The model under review builds one solid part; all positions refer to its coordinate system, in mm. A direction names the side the tool comes from. Give positions to 0.01 mm unless a question says otherwise; leave off trailing zeros. Order: outer loops, then holes, each group sorted by start corner. A loop starts at its lowest first (then second) coordinate and runs counter-clockwise, first axis right, second up. Notation, with made-up numbers: (26.25, 66.25) -> (33.25, 66.25) arc R27 ccw to (33.25, 89.25) -> close; hole circle Ø8 at (2, 19). An arc over 180 degrees is marked (long way). Use one line per item in the form item = value.
```python
from build123d import *

# Parameters (mm, degrees)
SKETCH1_W           = 70
SKETCH1_H           = 20
BOSS_EXTRUDE2_DEPTH = 3
SKETCH3_W           = 3
SKETCH3_H           = 20
BOSS_EXTRUDE3_DEPTH = 18
SKETCH4_W           = 46
SKETCH4_H           = 20
BOSS_EXTRUDE4_DEPTH = 3
SKETCH5_W           = 40
SKETCH5_H           = 3
CUT_EXTRUDE2_DEPTH  = 47.914816423
SKETCH6_R           = 3.1
CUT_EXTRUDE3_DEPTH  = 43.023802779
FILLET2_R           = 3
SKETCH7_R           = 1.6
CUT_EXTRUDE4_DEPTH  = 44.600458713
CUT_EXTRUDE5_DEPTH  = 26
SKETCH10_W          = 46
SKETCH10_H          = 20
BOSS_EXTRUDE5_DEPTH = 3
SKETCH11_R          = 3.1
CUT_EXTRUDE6_DEPTH  = 3
FILLET3_R           = 3


with BuildPart() as part:
    # Sketch1 → Boss-Extrude2 (new body)
    with BuildSketch(Plane(origin=(0, 0, 0), x_dir=(1, 0, 0), z_dir=(0, 1, 0))):
        Rectangle(SKETCH1_W, SKETCH1_H)
    extrude(amount=BOSS_EXTRUDE2_DEPTH)

    # Sketch3 → Boss-Extrude3 (add)
    with BuildSketch(Plane(origin=(0, 3, 0), x_dir=(1, 0, 0), z_dir=(0, 1, 0))):
        with Locations((21.5, 0)):
            Rectangle(SKETCH3_W, SKETCH3_H)
        with Locations((-21.5, 0)):
            Rectangle(SKETCH3_W, SKETCH3_H)
    extrude(amount=BOSS_EXTRUDE3_DEPTH)

    # Sketch4 → Boss-Extrude4 (add)
    with BuildSketch(Plane(origin=(0, 21, 0), x_dir=(1, 0, 0), z_dir=(0, 1, 0))):
        Rectangle(SKETCH4_W, SKETCH4_H)
    extrude(amount=BOSS_EXTRUDE4_DEPTH)

    # Sketch5 → Cut-Extrude2 (cut, through all)
    with BuildSketch(Plane.XY.offset(10)):
        with Locations((0, 1.5)):
            Rectangle(SKETCH5_W, SKETCH5_H)
    extrude(amount=-CUT_EXTRUDE2_DEPTH, mode=Mode.SUBTRACT)

    # Sketch6 → Cut-Extrude3 (cut, through all)
    with BuildSketch(Plane.XZ.offset(-21)):
        with Locations(Location((0, 0, 0), (0, 0, 270))):
            Circle(SKETCH6_R)
    extrude(amount=-CUT_EXTRUDE3_DEPTH, mode=Mode.SUBTRACT)

    # Fillet2
    fillet2_edges = [part.edges().sort_by_distance(p)[0] for p in [
        (-23, 24, 0),
        (23, 24, 0),
        (35, 1.5, 10),
        (-35, 1.5, 10),
        (-35, 1.5, -10),
        (35, 1.5, -10),
    ]]
    fillet(fillet2_edges, radius=FILLET2_R)

    # Sketch7 → Cut-Extrude4 (cut, through all)
    with BuildSketch(Plane.XZ):
        with Locations(Location((-27.499620905, -0.010826829, 0), (0, 0, 270))):
            Circle(SKETCH7_R)
        with Locations(Location((27.500379095, -0.010826829, 0), (0, 0, 270))):
            Circle(SKETCH7_R)
    extrude(amount=-CUT_EXTRUDE4_DEPTH, mode=Mode.SUBTRACT)

    # Sketch9 → Cut-Extrude5 (cut)
    with BuildSketch(Plane.XY.offset(10)):
        Polygon((0, 15.5), (-23, 15.5), (-23, 32.171258166), (25.72707431, 32.171258166), (25.72707431, 15.5), align=None)
    extrude(amount=-CUT_EXTRUDE5_DEPTH, mode=Mode.SUBTRACT)


with BuildPart() as cut_extrude5_piece_1:
    # of the separate pieces the step leaves, piece 1, a body of its own (cut_extrude5_pieces)
    add(part.part.solids().sort_by_distance((20, 15.5, 10))[0])



with BuildPart() as cut_extrude5_piece_2:
    # of the separate pieces the step leaves, piece 2, a body of its own (cut_extrude5_pieces)
    add(part.part.solids().sort_by_distance((-32, 0, 10))[0])


with BuildPart() as cut_extrude5_piece_1_1:
    add(cut_extrude5_piece_1.part)

    add(cut_extrude5_piece_2.part)  # Boss-Extrude5 merges Cut-Extrude5 piece 2
    # Sketch10 → Boss-Extrude5 (add)
    with BuildSketch(Plane(origin=(0, 15.5, 0), x_dir=(1, 0, 0), z_dir=(0, 1, 0))):
        Rectangle(SKETCH10_W, SKETCH10_H)
    extrude(amount=BOSS_EXTRUDE5_DEPTH)

    # Sketch11 → Cut-Extrude6 (cut)
    with BuildSketch(Plane(origin=(0, 18.5, 0), x_dir=(1, 0, 0), z_dir=(0, 1, 0))):
        with Locations(Location((0, 0, 0), (0, 0, 270))):
            Circle(SKETCH11_R)
    extrude(amount=-CUT_EXTRUDE6_DEPTH, mode=Mode.SUBTRACT)

    # Fillet3
    fillet3_edges = [cut_extrude5_piece_1_1.edges().sort_by_distance(p)[0] for p in [
        (-23, 18.5, 0),
        (23, 18.5, 0),
    ]]
    fillet(fillet3_edges, radius=FILLET3_R)


solid = cut_extrude5_piece_1_1.part
```
1. Add section D-D on z = 4.25. Give the boundary of the cut face in (x, y), then the cut area to 3 significant figures.
Values:
outline = (-35, 0) -> (-20, 0) -> (-20, 15.5) -> (20, 15.5) -> (20, 0) -> (35, 0) -> (35, 3) -> (23, 3) -> (23, 15.5) arc R3 ccw to (20, 18.5) -> (-20, 18.5) arc R3 ccw to (-23, 15.5) -> (-23, 3) -> (-35, 3) -> close
area = 299 mm^2
2. Add section B-B on x = 0. Give the boundary of the cut face in (y, z), then the cut area to 3 significant figures.
Values:
outline = (15.5, -10) -> (18.5, -10) -> (18.5, -3.1) -> (15.5, -3.1) -> close; (15.5, 3.1) -> (18.5, 3.1) -> (18.5, 10) -> (15.5, 10) -> close
area = 41.4 mm^2
3. Add section A-A on y = 6.75. Give the boundary of the cut face in (x, z).
Values:
outline = (-23, -10) -> (-20, -10) -> (-20, 10) -> (-23, 10) -> close; (20, -10) -> (23, -10) -> (23, 10) -> (20, 10) -> close
4. Add section C-C on z = 0. Give the boundary of the cut face in (x, y), then the cut area to 3 significant figures.
Values:
outline = (-35, 0) -> (-29.1, 0) -> (-29.1, 3) -> (-35, 3) -> close; (-25.9, 0) -> (-20, 0) -> (-20, 15.5) -> (-3.1, 15.5) -> (-3.1, 18.5) -> (-20, 18.5) arc R3 ccw to (-23, 15.5) -> (-23, 3) -> (-25.9, 3) -> close; (3.1, 15.5) -> (20, 15.5) -> (20, 0) -> (25.9, 0) -> (25.9, 3) -> (23, 3) -> (23, 15.5) arc R3 ccw to (20, 18.5) -> (3.1, 18.5) -> close; (29.1, 0) -> (35, 0) -> (35, 3) -> (29.1, 3) -> close
area = 261 mm^2
5. The part is to be moulded in two halves that separate along X. For faces 1 (the face through (-28.47, 1.48, 1.26)), 2 (the face through (25.94, 1.48, 0.34)), 3 (the face through (-35, 1, 0)), 4 (the face through (34.1, 1.52, 9.14)), say which applies: +X half, -X half, draft (parallel to the pull), parting line (faces both ways), or undercut.
Values:
face_1 = undercut
face_2 = undercut
face_3 = -X half
face_4 = +X half
6. For L1, parallel to X at y = 8, z = 1; L2, parallel to X at y = 2.5, z = -3.75; L3, parallel to Y at x = -9.5, z = 5.5, list the stretches that pass through material, from the lowest coordinate up.
Values:
L1 = -23 to -20, 20 to 23
L2 = -35 to -20, 20 to 35
L3 = 15.5 to 18.5
7. Tool access review of faces 5 (the face through (-30, 3, 0)), 6 (the face through (34.1, 1.52, -9.14)), 7 (the face through (-20, 8, 0)), 8 (the face through (23, 9, 0)): name each direction out of +Z, -Z, +X, -X, +Y, -Y from which nothing blocks a thin tool from reaching the whole face with its end or side.
Values:
face_5 = +Z, -Z, -X, +Y
face_6 = -Z, +X, +Y, -Y
face_7 = +Z, -Z, -Y
face_8 = +Z, -Z, +X, +Y
8. For pin 1 Ø3 at (x, z) = (1.5, -4) entering from -Y; pin 2 Ø8 at (y, z) = (7.5, 3) entering from -X; pin 3 Ø9.5 at (x, z) = (30.5, 3.5) entering from +Y, all flat-tipped, find the tip position at first contact; note any pin that passes through.
Values:
pin_1 = 15.5
pin_2 = -23
pin_3 = 3
